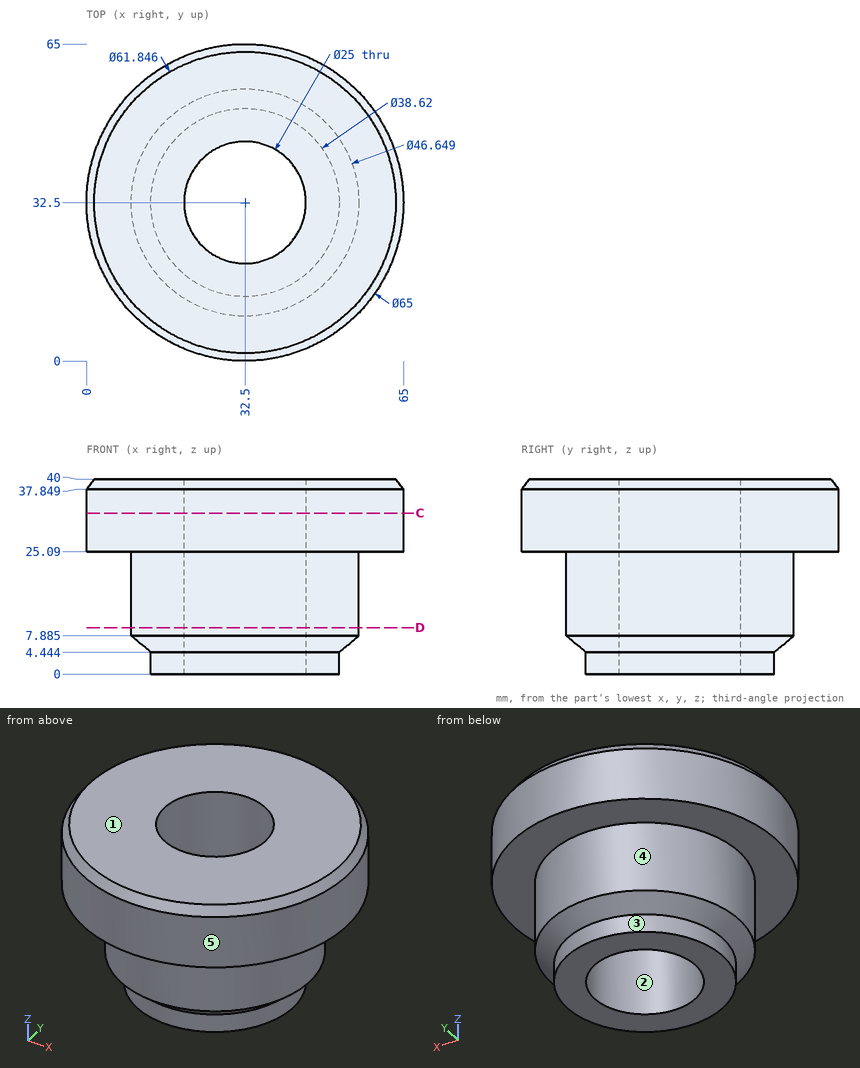
Print and shaded views of the part. All mm, measured from the part's lowest x, y and z. A direction names the side the tool comes from. Give positions to 0.01 mm unless a question says otherwise; leave off trailing zeros. Order: outer loops, then holes, each group sorted by start corner. A loop starts at its lowest first (then second) coordinate and runs counter-clockwise, first axis right, second up. Notation, with made-up numbers: (-13.5, -1) - (8.5, -1) arc R20 cw to (8.5, 19) - close; hole circle Ø7 at (-10, 81.5). An arc over 180 degrees is marked (long way). One line per item, written item: value.
Item 1: Pin check, flat tips, straight feed: pin 1 Ø22.5 at (x, y) = (32.5, 32.5) entering from +Z; pin 2 Ø3 at (x, y) = (36.5, 52) entering from -Z; pin 3 Ø1 at (y, z) = (25, 31) entering from -X; pin 4 Ø1.5 at (x, y) = (17, 52.5) entering from -Z. Stop position of each tip, or through.
Response values:
pin 1: through
pin 2: z = 0
pin 3: x = 0.76
pin 4: z = 25.09
Item 2: Slice it at C-C (z = 33). List the corners of the cut face in (x, y).
Response values:
outline: circle Ø65 at (32.5, 32.5); hole circle Ø25 at (32.5, 32.5)
Item 3: Two-plate mould, pull along Y, no slides. Class the marked faces 1, 2 and 3: released by +Y, released by -Y, zero draft, split by the parting line, or undercut.
Response values:
face 1: zero draft
face 2: undercut
face 3: split by the parting line
Item 4: Tool access for the marked faces 4 and 5: list every direction of +Z, -Z, +X, -X, +Y, -Y with a clear straight run to the whole face (end or side of a thin tool).
Response values:
face 4: -Z
face 5: +Z, -Z
Item 5: Wall check: line 1 (Y direction, x = 32.5, z = 19.5) (1 decimal); line 2 (X direction, y = 32, z = 28). Give the ranges that are in metal, low to high.
Response values:
line 1: 9.2 to 20, 45 to 55.8
line 2: 0 to 20.01, 44.99 to 65
Item 6: Slice it at D-D (z = 9.5). List the corners of the cut face in (x, y) (1 decimal).
Response values:
outline: circle Ø46.6 at (32.5, 32.5); hole circle Ø25 at (32.5, 32.5)
